```python
from build123d import *

# Parameters (mm, degrees)
SKETCH1_R           = 25
SKETCH1_R_2         = 2.5
SKETCH1_R_3         = 10
BOSS_EXTRUDE1_DEPTH = 5
SKETCH2_R           = 12.5
BOSS_EXTRUDE2_DEPTH = 20
SKETCH3_R           = 7.5
BOSS_EXTRUDE3_DEPTH = 17.5
SKETCH4_R           = 2.4
CUT_EXTRUDE1_DEPTH  = 10


with BuildPart() as part:
    # Sketch1 → Boss-Extrude1 (new body)
    # profile 1 of 2: a face of its own
    with BuildSketch(Plane.XY):
        Circle(SKETCH1_R)
        with Locations((-17.5, 0)):
            Circle(SKETCH1_R_2, mode=Mode.SUBTRACT)
        with Locations((0, -17.5)):
            Circle(SKETCH1_R_2, mode=Mode.SUBTRACT)
        with Locations((17.5, 0)):
            Circle(SKETCH1_R_2, mode=Mode.SUBTRACT)
        with Locations((0, 17.5)):
            Circle(SKETCH1_R_2, mode=Mode.SUBTRACT)
        Circle(SKETCH1_R_3, mode=Mode.SUBTRACT)
    # profile 2 of 2: a face of its own
    with BuildSketch(Plane.XY):
        Circle(SKETCH1_R_3)
    extrude(amount=BOSS_EXTRUDE1_DEPTH)

    # Sketch2 → Boss-Extrude2 (add)
    with BuildSketch(Plane.XY.offset(5)):
        Circle(SKETCH2_R)
    extrude(amount=BOSS_EXTRUDE2_DEPTH)

    # Sketch3 → Boss-Extrude3 (add)
    with BuildSketch(Plane.XY.offset(25)):
        Circle(SKETCH3_R)
    extrude(amount=BOSS_EXTRUDE3_DEPTH)

    # Sketch4 → Cut-Extrude1 (cut)
    with BuildSketch(Plane.XY.offset(42.5)):
        Circle(SKETCH4_R)
    extrude(amount=-CUT_EXTRUDE1_DEPTH, mode=Mode.SUBTRACT)


solid = part.part
```
Source: CAD feature listing. Evaluate the final solid. Frame: model axes, mm. A direction names the side the tool comes from. Give positions to 0.01 mm unless a question says otherwise; leave off trailing zeros. Order: outer loops, then holes, each group sorted by start corner. A loop starts at its lowest first (then second) coordinate and runs counter-clockwise, first axis right, second up. Notation, with made-up numbers: (58, -3) -> (110, -3) arc R13 ccw to (110, 12) -> close; hole circle Ø11 at (2.25, 52). An arc over 180 degrees is marked (long way). Use a Markdown table: item, result.
Q1. First-contact query: P1, Ø4.5, axis at x = 0, y = 0, coming from the +Z side; P2, Ø4, axis at x = -18.5, y = 9.5, coming from the +Z side; P3, Ø5, axis at x = -10.5, z = 13.5, coming from the +Y side. Flat tips, straight axial feed; report the tip coordinate or a pass-through.
A:
| item | result |
|---|---|
| P1 | z = 32.5 |
| P2 | z = 5 |
| P3 | y = 9.6 |
Q2. Section D-D (y = -19). Return the cut outline in (x, z), and give its area (3 significant figures).
A:
| item | result |
|---|---|
| outline | (-16.25, 0) -> (-2, 0) -> (-2, 5) -> (-16.25, 5) -> close; (2, 0) -> (16.25, 0) -> (16.25, 5) -> (2, 5) -> close |
| area | 142 mm^2 |
Q3. Section A-A (y = 0). Return the cut outline in (x, z), and give its area (4 significant figures).
A:
| item | result |
|---|---|
| outline | (-25, 0) -> (-20, 0) -> (-20, 5) -> (-25, 5) -> close; (-15, 0) -> (15, 0) -> (15, 5) -> (12.5, 5) -> (12.5, 25) -> (7.5, 25) -> (7.5, 42.5) -> (2.4, 42.5) -> (2.4, 32.5) -> (-2.4, 32.5) -> (-2.4, 42.5) -> (-7.5, 42.5) -> (-7.5, 25) -> (-12.5, 25) -> (-12.5, 5) -> (-15, 5) -> close; (20, 0) -> (25, 0) -> (25, 5) -> (20, 5) -> close |
| area | 914.5 mm^2 |
Q4. Material intervals for line 1 (Y direction, x = 0, z = 1.85); line 2 (Y direction, x = 0, z = 37); line 3 (Z direction, x = 21, y = -8), sorted ascending. Write a range as [from, to].
A:
| item | result |
|---|---|
| line 1 | [-25, -20], [-15, 15], [20, 25] |
| line 2 | [-7.5, -2.4], [2.4, 7.5] |
| line 3 | [0, 5] |
Q5. Access query for faces 1 (the face through (0, 0, 32.5)), 2 (the face through (15, 0, 2)). Directions: +Z, -Z, +X, -X, +Y, -Y. A direction counts if a zero-diameter tool reaches every point of the face in a straight line with its end or side. Return the directions, or none.
A:
| item | result |
|---|---|
| face 1 | +Z |
| face 2 | +Z, -Z |
Q6. Section C-C (x = 17.5). Return the cut outline in (y, z), and give its area (3 significant figures).
A:
| item | result |
|---|---|
| outline | (-17.85, 0) -> (-2.5, 0) -> (-2.5, 5) -> (-17.85, 5) -> close; (2.5, 0) -> (17.85, 0) -> (17.85, 5) -> (2.5, 5) -> close |
| area | 154 mm^2 |
Q7. Pull-direction query (X, two-part tool) for faces 3 (the face through (0, -8, 25)), 4 (the face through (11.923, 3.755, 14.86)), 5 (the face through (-0.54, -19.94, 2.46)); classes: +X half, -X half, draft (parallel to the pull), parting line (faces both ways), or undercut.
A:
| item | result |
|---|---|
| face 3 | draft |
| face 4 | parting line |
| face 5 | undercut |
